from build123d import *

# Parameters (mm, degrees)
BASES_R             = 6.35
BASE_DEPTH          = 7.3
HORN_HALF_DEPTH     = 2.5
TOOTH_DEPTH         = 3
TOOTH_CP_COUNT      = 26
BOTTOM_START        = -3
BOTTOMBORES_R       = 2.7
BOTTOM_BORE_DEPTH   = 3
HOLDINGSHAFTS_R     = 6.35
HOLDINGSHAFTS_R_2   = 4.25
HOLDING_SHAFT_DEPTH = 4.8
HORNATTACHS_R       = 1.25
CUT_EXTRUDE_1_DEPTH = 8.3
TOPBORES_R          = 1.6
CUT_EXTRUDE_2_DEPTH = 8.3


with BuildPart() as part:
    # BaseS → BASE (new body)
    with BuildSketch(Plane(origin=(0, 0, 0), x_dir=(1, 0, 0), z_dir=(0, 1, 0))):
        Circle(BASES_R)
    extrude(amount=BASE_DEPTH)

    # HornHalfS → HORN HALF (add)
    with BuildSketch(Plane(origin=(0, 7.3, 0), x_dir=(1, 0, 0), z_dir=(0, 1, 0))):
        with BuildLine():
            Line((-2.609740545, 12.460167671), (-3.926899835, 4.990186137))
            ThreePointArc((-3.926899835, 4.990186137), (0, 6.35), (3.926899835, 4.990186137))
            Line((3.926899835, 4.990186137), (2.609740545, 12.460167671))
            ThreePointArc((2.609740545, 12.460167671), (0, 14.65), (-2.609740545, 12.460167671))
        make_face()
    extrude(amount=-HORN_HALF_DEPTH)

    # ToothS → TOOTH (cut)
    with BuildSketch(Plane.XZ):
        with BuildLine():
            Line((0, -3), (0.262459231, -2.687213269))
            ThreePointArc((0.262459231, -2.687213269), (0, -2.7), (-0.262459231, -2.687213269))
            Line((-0.262459231, -2.687213269), (0, -3))
        make_face()
    tooth = extrude(amount=-TOOTH_DEPTH, mode=Mode.SUBTRACT)

    # TOOTH CP: TOOTH ×26 about axis
    tooth_cp_axis = Axis((0, 0, 0), (0, 1, 0))
    for i in range(1, TOOTH_CP_COUNT):
        add(tooth.rotate(tooth_cp_axis, i * 360 / TOOTH_CP_COUNT), mode=Mode.SUBTRACT)

    # BottomBoreS → BOTTOM BORE (cut)
    with BuildSketch(Plane(origin=(0, 0, 0), x_dir=(-1, 0, 0), z_dir=(0, -1, 0)).offset(BOTTOM_START)):
        Circle(BOTTOMBORES_R)
    extrude(amount=BOTTOM_BORE_DEPTH, mode=Mode.SUBTRACT)

    # HoldingShaftS → HOLDING SHAFT (cut)
    with BuildSketch(Plane.XZ):
        Circle(HOLDINGSHAFTS_R)
        Circle(HOLDINGSHAFTS_R_2, mode=Mode.SUBTRACT)
    extrude(amount=-HOLDING_SHAFT_DEPTH, mode=Mode.SUBTRACT)

    # HornAttachS → 除料-伸長1 (cut, through all)
    with BuildSketch(Plane(origin=(0, 7.3, 0), x_dir=(1, 0, 0), z_dir=(0, 1, 0))):
        with Locations((0, 12)):
            Circle(HORNATTACHS_R)
    extrude(amount=-CUT_EXTRUDE_1_DEPTH, mode=Mode.SUBTRACT)

    # TopBoreS → 除料-伸長2 (cut, through all)
    with BuildSketch(Plane(origin=(0, 7.3, 0), x_dir=(1, 0, 0), z_dir=(0, 1, 0))):
        Circle(TOPBORES_R)
    extrude(amount=-CUT_EXTRUDE_2_DEPTH, mode=Mode.SUBTRACT)


solid = part.part
Read the model definition and answer for the solid it produces. Units are mm, in the model's axes. A direction names the side the tool comes from. Coordinates: 2 decimals unless noted, no trailing zeros. Loops run counter-clockwise (first coordinate to the right, second up) from the corner with the lowest first, then second, coordinate; pieces in that order, holes last. Notation, with made-up numbers: (29, 6) -> (41, 6) arc R24 cw to (41, 18) -> close; hole circle Ø8 at (45.5, -19). An arc over 180 degrees is marked (long way). Answer in a Markdown table with one row per item.
Item 1: For a pull along X with two mould halves and no side action, classify faces 1 (the flat face through (3, 0, 0)), 2 (the cylindrical face through (-1.27, 5.18, 0.97)), 3 (the cylindrical face through (0.05, 6.07, -14.65)) as released by +X, released by -X, zero draft, split by the parting line, or undercut.
Returned:
| item | result |
|---|---|
| face 1 | zero draft |
| face 2 | undercut |
| face 3 | split by the parting line |
Item 2: Each of these flat-tipped pins is pushed along its axis until it touches: P1, Ø1.5, axis at y = 5.5, z = -12.5, coming from the -X side; P2, Ø1.5, axis at y = 2.5, z = -0.5, coming from the +X side; P3, Ø3, axis at x = 1, z = -0.5, coming from the -Y side. Where does it stop, or does it pass through?
Returned:
| item | result |
|---|---|
| P1 | stops at x = -2.73 |
| P2 | stops at x = 4.25 |
| P3 | stops at y = 3 |
Item 3: A cutting plane is placed at A-A on y = 6.25. Determine the outline of the cut face in (x, z), plus the area to 3 significant figures.
Returned:
| item | result |
|---|---|
| outline | (-3.93, -4.99) -> (-2.61, -12.46) arc R2.65 ccw to (2.61, -12.46) -> (3.93, -4.99) arc R6.35 ccw (long way) to start; hole circle Ø3.2 at (0, 0); hole circle Ø2.5 at (0, -12) |
| area | 164 mm^2 |
Item 4: Straight lines are drawn through the part: line 1 along Z through (x, y) = (0, 6.3); line 2 along Z through (x, y) = (-1, 5); line 3 along X through (y, z) = (5, 0). For each, find the intervals that lie inside material, in ascending order. Write a range as [from, to].
Returned:
| item | result |
|---|---|
| line 1 | z = [-14.65, -13.25], [-10.75, -1.6], [1.6, 6.35] |
| line 2 | z = [-14.45, -12.75], [-11.25, -1.25], [1.25, 6.27] |
| line 3 | x = [-6.35, -1.6], [1.6, 6.35] |
Item 5: For faces 4 (the flat face through (-1.3, 3, 1.3)), 5 (the cylindrical face through (-0.22, 6.032, 6.346)), determine the directions among +Z, -Z, +X, -X, +Y, -Y from which every point of the face is accessible in a straight line to the end or side of a thin tool.
Returned:
| item | result |
|---|---|
| face 4 | -Y |
| face 5 | +Y, -Y |
Item 6: A cutting plane is placed at C-C on y = 4. Determine the outline of the cut face in (x, z), plus the area to 3 significant figures.
Returned:
| item | result |
|---|---|
| outline | circle Ø8.5 at (0, 0); hole circle Ø3.2 at (0, 0) |
| area | 48.7 mm^2 |
Item 7: A cutting plane is placed at B-B on z = -12. Determine the outline of the cut face in (x, y).
Returned:
| item | result |
|---|---|
| outline | (-2.69, 4.8) -> (-1.25, 4.8) -> (-1.25, 7.3) -> (-2.69, 7.3) -> close; (1.25, 4.8) -> (2.69, 4.8) -> (2.69, 7.3) -> (1.25, 7.3) -> close |
Item 8: A cutting plane is placed at D-D on z = -3.5. Determine the outline of the cut face in (x, y), plus the area to 3 significant figures.
Returned:
| item | result |
|---|---|
| outline | (-5.3, 4.8) -> (-2.41, 4.8) -> (-2.41, 0) -> (2.41, 0) -> (2.41, 4.8) -> (5.3, 4.8) -> (5.3, 7.3) -> (-5.3, 7.3) -> close |
| area | 49.6 mm^2 |
